Autodesk Inventor part; units mm, degrees
ref_plane "YZ Plane" through (0, 0, 0) normal (1, 0, 0) x (0, 1, 0)
ref_plane "XZ Plane" through (0, 0, 0) normal (0, 1, 0) x (-1, 0, 0)
ref_plane "XY Plane" through (0, 0, 0) normal (0, 0, 1) x (1, 0, 0)
sketch "Sketch1" plane through (0, 0, 0) normal (0, 1, 0) x (-1, 0, 0)
  line L0 (6.35, 0) -> (209.55, 0)
  line L1 (215.9, -6.35) -> (215.9, -6.35)
  circle A0 centre (6.35, -6.35) radius 2.1844
  circle A1 centre (209.55, -6.35) radius 2.1844
  line L2 (38.1, -19.05) -> (38.1, -69.85)
  line L3 (215.9, -82.55) -> (215.9, -82.55)
  line L4 (209.55, -88.9) -> (6.35, -88.9)
  line L5 (0, -82.55) -> (0, -82.55)
  line L6 (50.8, -19.05) -> (50.8, -69.85)
  line L7 (209.55, -12.7) -> (57.15, -12.7)
  line L8 (31.75, -12.7) -> (6.35, -12.7)
  line L9 (6.35, -76.2) -> (31.75, -76.2)
  line L10 (57.15, -76.2) -> (209.55, -76.2)
  arc A2 (57.15, -12.7) -> (50.8, -19.05) centre (57.15, -19.05) ccw
  arc A3 (38.1, -19.05) -> (31.75, -12.7) centre (31.75, -19.05) ccw
  arc A4 (31.75, -76.2) -> (38.1, -69.85) centre (31.75, -69.85) ccw
  arc A5 (50.8, -69.85) -> (57.15, -76.2) centre (57.15, -69.85) ccw
  line L11 (0, -6.35) -> (0, -6.35)
  line L12 (0, -76.2) -> (0, -88.9)
  circle A6 centre (209.55, -82.55) radius 2.1844
  circle A7 centre (6.35, -82.55) radius 2.1844
  arc A8 (215.9, -6.35) -> (209.55, 0) centre (209.55, -6.35) ccw
  arc A9 (209.55, -12.7) -> (215.9, -6.35) centre (209.55, -6.35) ccw
  arc A10 (0, -6.35) -> (6.35, -12.7) centre (6.35, -6.35) ccw
  arc A11 (6.35, 0) -> (0, -6.35) centre (6.35, -6.35) ccw
  arc A12 (6.35, -76.2) -> (0, -82.55) centre (6.35, -82.55) ccw
  arc A13 (0, -82.55) -> (6.35, -88.9) centre (6.35, -82.55) ccw
  arc A14 (215.9, -82.55) -> (209.55, -76.2) centre (209.55, -82.55) ccw
  arc A15 (209.55, -88.9) -> (215.9, -82.55) centre (209.55, -82.55) ccw
  point P0 (0, 0)
  point P1 (215.9, 0)
  point P2 (215.9, -12.7)
  point P3 (0, -12.7)
  point P4 (38.1, -12.7)
  point P5 (38.1, -76.2)
  point P6 (215.9, -76.2)
  point P7 (215.9, -88.9)
  dimension "d0" = 215.9
  dimension "d1" = 12.7
  dimension "d2" = 4.3688
  dimension "d3" = 63.5
  dimension "d4" = 12.7
  dimension "d5" = 12.7
  dimension "d6" = 38.1
  dimension "d7" = 6.35
  dimension "d8" = 6.35
extrude "Extrusion1" add sketch "Sketch1" along normal blind 1.5875
properties part number "Ring Guardd"
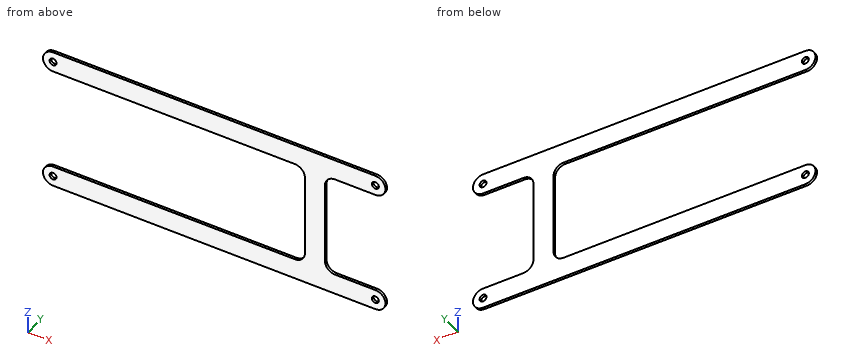
Geometry: final body of the model. Coordinates: model frame, mm. Round coordinates to 2 decimals unless told otherwise and drop trailing zeros. Order: outer loops, then holes, each group sorted by start corner. A loop starts at its lowest first (then second) coordinate and runs counter-clockwise, first axis right, second up. Notation, with made-up numbers: (-10.5, -1) -> (-1.5, -1) arc R18 ccw to (-1.5, 24) -> close; hole circle Ø2 at (67, -25). An arc over 180 degrees is marked (long way). Put each result on its own line as item: value. Start each with the question number.
Q1. Section C-C on y = 1.3. Return the cut outline in (x, z), and give its area (3 significant figures).
Q2. First-contact query: pin 1 (0.5 mm diameter, centred on y = 1, z = -43.5, fed in from -X); pin 2 (5 mm diameter, centred on x = -209.55, z = -82.55, fed in from +Y); pin 3 (0.5 mm diameter, centred on y = 1, z = -46, fed in from +X). Flat tips, straight axial feed; report the tip coordinate or a pass-through.
Q3. Section A-A on x = -202. Return the cut outline in (y, z).
Q4. Section D-D on z = -54.5. Return the cut outline in (x, y), and give its area (3 significant figures).
Q5. Section B-B on z = -6.35. Return the cut outline in (x, y).
Q6. Line query: probe 1 along X at (y, z) = (0.55, -82.5); probe 2 along Z at (x, y) = (-209.55, 0.3); probe 3 along Z at (x, y) = (-74, 1.2). Output: solid intervals per line, ascending.
Ans:
1. outline: (-209.55, -88.9) -> (-6.35, -88.9) arc R6.35 ccw to (-6.35, -76.2) -> (-31.75, -76.2) arc R6.35 cw to (-38.1, -69.85) -> (-38.1, -19.05) arc R6.35 cw to (-31.75, -12.7) -> (-6.35, -12.7) arc R6.35 ccw to (-6.35, 0) -> (-209.55, 0) arc R6.35 ccw to (-209.55, -12.7) -> (-57.15, -12.7) arc R6.35 cw to (-50.8, -19.05) -> (-50.8, -69.85) arc R6.35 cw to (-57.15, -76.2) -> (-209.55, -76.2) arc R6.35 ccw to start; hole circle Ø4.37 at (-209.55, -82.55); hole circle Ø4.37 at (-209.55, -6.35); hole circle Ø4.37 at (-6.35, -82.55); hole circle Ø4.37 at (-6.35, -6.35)
1. area: 6,200 mm2
2. pin 1: stops at x = -50.8
2. pin 2: stops at y = 1.59
2. pin 3: stops at x = -38.1
3. outline: (0, -88.9) -> (1.59, -88.9) -> (1.59, -76.2) -> (0, -76.2) -> close; (0, -12.7) -> (1.59, -12.7) -> (1.59, 0) -> (0, 0) -> close
4. outline: (-50.8, 0) -> (-38.1, 0) -> (-38.1, 1.59) -> (-50.8, 1.59) -> close
4. area: 20.2 mm2
5. outline: (-215.9, 0) -> (-211.73, 0) -> (-211.73, 1.59) -> (-215.9, 1.59) -> close; (-207.37, 0) -> (-8.53, 0) -> (-8.53, 1.59) -> (-207.37, 1.59) -> close; (-4.17, 0) -> (0, 0) -> (0, 1.59) -> (-4.17, 1.59) -> close
6. probe 1: x = -215.9 to -211.73, -207.37 to -8.53, -4.17 to 0
6. probe 2: z = -88.9 to -84.73, -80.37 to -76.2, -12.7 to -8.53, -4.17 to 0
6. probe 3: z = -88.9 to -76.2, -12.7 to 0
